The listing builds one solid part. Answer for the finished solid, in the listing's coordinates (mm). Face numbers are marked on the shaded views. A direction names the side the tool comes from. Round coordinates to 2 decimals unless told otherwise and drop trailing zeros. Order: outer loops, then holes, each group sorted by start corner. A loop starts at its lowest first (then second) coordinate and runs counter-clockwise, first axis right, second up. Notation, with made-up numbers: (86, 60.25) -> (111, 60.25) arc R26 cw to (111, 77.25) -> close; hole circle Ø10 at (35.25, -21.5). An arc over 180 degrees is marked (long way). Return JSON: item names as keys, results as strings. Group by question number.
(1) Consider line 1 (Z direction, x = -5, y = 4.25); line 2 (X direction, y = 1.75, z = -8); line 3 (Z direction, x = 16.5, y = 3.5). Determine where each line is inside the solid, lowest interval first. Write a range as [from, to].
(2) The part is cut by section B-B (x = 0). Determine the outline of the cut face in (y, z).
(3) Which of the six approach directions +Z, -Z, +X, -X, +Y, -Y give full straight-line access (tool end or side, diameter ignored) to the marked faces 1 and 2?
(4) This flat-tipped pin is pushed along its axis until it touches: pin 1 (3.5 mm diameter, centred on x = -11, z = -8, fed in from +Y). Where does it stop, or does it pass through?
(5) The part is cut by section C-C (x = 13). Determine the outline of the cut face in (y, z).
(6) The part is cut by section D-D (z = -12.7). Determine the outline of the cut face in (x, y).
(7) The part is cut by section A-A (y = 4.25). Determine the outline of the cut face in (x, z), plus the area to 3 significant figures.
(8) Determine the mould class of the marked faces 3, 4 and 5 for opening direction Z: +Z half, -Z half, draft (parallel to the pull), parting line (faces both ways), or undercut.
from build123d import *

# Parameters (mm, degrees)
SKETCH1_W               = 49.784
SKETCH1_H               = 50.8
BOSS_EXTRUDE1_DEPTH     = 6.35
F_8_CLEARANCE_HOLE1_D   = 4.4958
F_1_4_CLEARANCE_HOLE1_D = 6.7564
CUT_EXTRUDE1_DEPTH      = 4.064
SKETCH9_R               = 2.38125
CUT_EXTRUDE2_DEPTH      = 37.126087029
BODY_MOVE_COPY1_ANGLE   = 180


with BuildPart() as part:
    # Sketch1 → Boss-Extrude1 (new body)
    with BuildSketch(Plane(origin=(0, 0, 0), x_dir=(1, 0, 0), z_dir=(0, 1, 0))):
        Rectangle(SKETCH1_W, SKETCH1_H)
    extrude(amount=BOSS_EXTRUDE1_DEPTH)

    # #8 Clearance Hole1 (through all)
    with Locations(Plane(origin=(0, 6.35, 0), x_dir=(1, 0, 0), z_dir=(0, 1, 0))):
        with Locations((-18.288, 12.7), (18.288, 12.7), (0, -12.7)):
            Hole(F_8_CLEARANCE_HOLE1_D / 2)

    # 1/4 Clearance Hole1 (through all)
    with Locations(Plane(origin=(0, 6.35, 0), x_dir=(1, 0, 0), z_dir=(0, 1, 0))):
        with Locations((0, 14.61008), (-13.86078, -10.78992), (13.86078, -10.78992)):
            Hole(F_1_4_CLEARANCE_HOLE1_D / 2)

    # Sketch8 → Cut-Extrude1 (cut)
    with BuildSketch(Plane.XZ):
        with BuildLine():
            Line((-19.44878, 16.37792), (-19.44878, 5.20192))
            ThreePointArc((-19.44878, 5.20192), (-13.86078, -0.38608), (-8.27278, 5.20192))
            Line((-8.27278, 5.20192), (-8.27278, 16.37792))
            ThreePointArc((-8.27278, 16.37792), (-13.86078, 21.96592), (-19.44878, 16.37792))
        make_face()
        with BuildLine():
            Line((8.27278, 16.37792), (8.27278, 5.20192))
            ThreePointArc((8.27278, 5.20192), (13.86078, -0.38608), (19.44878, 5.20192))
            Line((19.44878, 5.20192), (19.44878, 16.37792))
            ThreePointArc((19.44878, 16.37792), (13.86078, 21.96592), (8.27278, 16.37792))
        make_face()
        with BuildLine():
            Line((-5.588, -9.02208), (5.588, -9.02208))
            ThreePointArc((5.588, -9.02208), (11.176, -14.61008), (5.588, -20.19808))
            Line((5.588, -20.19808), (-5.588, -20.19808))
            ThreePointArc((-5.588, -20.19808), (-11.176, -14.61008), (-5.588, -9.02208))
        make_face()
    extrude(amount=-CUT_EXTRUDE1_DEPTH, mode=Mode.SUBTRACT)

    # Sketch9 → Cut-Extrude2 (cut, through all)
    with BuildSketch(Plane(origin=(0, 6.35, 0), x_dir=(1, 0, 0), z_dir=(0, 1, 0))):
        with Locations(Location((0, 0, 0), (0, 0, 270))):
            Circle(SKETCH9_R)
    extrude(amount=-CUT_EXTRUDE2_DEPTH, mode=Mode.SUBTRACT)


with BuildPart() as part_1:
    # Body-Move/Copy1: moved
    add(part.part.rotate(Axis((0, 3.175, 0), (1, 0, 0)), BODY_MOVE_COPY1_ANGLE))


solid = part_1.part
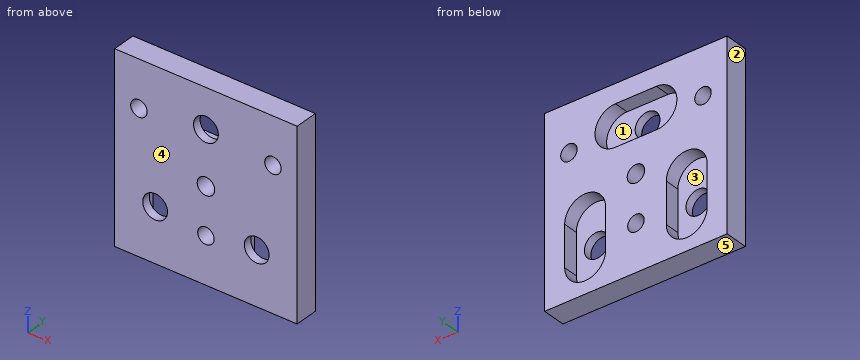
Answer below:
{
 "1": {"line 1": "z = [-25.4, 9.02], [20.2, 25.4]", "line 2": "x = [-24.89, -15.77], [-11.96, 11.96], [15.77, 24.89]", "line 3": "z = [-25.4, -21.3], [-0.28, 11.34], [14.06, 25.4]"},
 "2": {"outline": "(0, -25.4) -> (6.35, -25.4) -> (6.35, -14.95) -> (0, -14.95) -> close; (0, -10.45) -> (6.35, -10.45) -> (6.35, -2.38) -> (0, -2.38) -> close; (0, 2.38) -> (6.35, 2.38) -> (6.35, 9.02) -> (2.29, 9.02) -> (2.29, 11.23) -> (0, 11.23) -> close; (0, 17.99) -> (2.29, 17.99) -> (2.29, 20.2) -> (6.35, 20.2) -> (6.35, 25.4) -> (0, 25.4) -> close"},
 "3": {"face 1": "+Y", "face 2": "+Z, -Z, -X, +Y, -Y"},
 "4": {"pin 1": "stops at y = 2.29"},
 "5": {"outline": "(0, -25.4) -> (6.35, -25.4) -> (6.35, -21.9) -> (2.29, -21.9) -> (2.29, -14.06) -> (0, -14.06) -> close; (0, -7.52) -> (2.29, -7.52) -> (2.29, 0.32) -> (6.35, 0.32) -> (6.35, 25.4) -> (0, 25.4) -> close"},
 "6": {"outline": "(-24.89, 0) -> (-16.65, 0) -> (-16.65, 2.29) -> (-19.45, 2.29) -> (-19.45, 6.35) -> (-24.89, 6.35) -> close; (-11.07, 0) -> (-2.25, 0) -> (-2.25, 6.35) -> (-8.27, 6.35) -> (-8.27, 2.29) -> (-11.07, 2.29) -> close; (2.25, 0) -> (11.07, 0) -> (11.07, 2.29) -> (8.27, 2.29) -> (8.27, 6.35) -> (2.25, 6.35) -> close; (16.65, 0) -> (24.89, 0) -> (24.89, 6.35) -> (19.45, 6.35) -> (19.45, 2.29) -> (16.65, 2.29) -> close"},
 "7": {"outline": "(-24.89, -25.4) -> (24.89, -25.4) -> (24.89, 25.4) -> (-24.89, 25.4) -> close; hole circle Ø4.5 at (-18.29, 12.7); hole (-19.45, -16.38) arc R5.59 ccw to (-8.27, -16.38) -> (-8.27, -5.2) arc R5.59 ccw to (-19.45, -5.2) -> close; hole (-5.59, 9.02) -> (5.59, 9.02) arc R5.59 ccw to (5.59, 20.2) -> (-5.59, 20.2) arc R5.59 ccw to start; hole circle Ø4.76 at (0, 0); hole circle Ø4.5 at (0, -12.7); hole (8.27, -16.38) arc R5.59 ccw to (19.45, -16.38) -> (19.45, -5.2) arc R5.59 ccw to (8.27, -5.2) -> close; hole circle Ø4.5 at (18.29, 12.7)", "area": "1,790 mm²"},
 "8": {"face 3": "undercut", "face 4": "draft", "face 5": "-Z half"}
}
